Could you check a few things on this model? Use its own coordinates, in mm. Coordinates: 2 decimals unless noted, no trailing zeros. Write each loop counter-clockwise with the first axis right and the second up, starting at its lowest first coordinate (ties: lowest second). Pieces come first, ordered by that corner, then holes.
Item 1: I want a section at C-C on y = -323.5. Please give me the cut outline in (x, z), then the cut area to 3 significant figures.
Item 2: If I drill on probe 1 along Y at (x, z) = (-621, 1.3); probe 2 along X at (y, z) = (-349, 1.55); probe 3 along X at (y, z) = (-261, 1.55), over which ranges is the centre line in solid material (lowest first)?
Item 3: I want a section at A-A on z = 0.9. Please give me the cut outline in (x, y), then the cut area to 3 significant figures.
Item 4: I want a section at B-B on y = -208.5. Please give me the cut outline in (x, z), then the cut area to 3 significant figures.
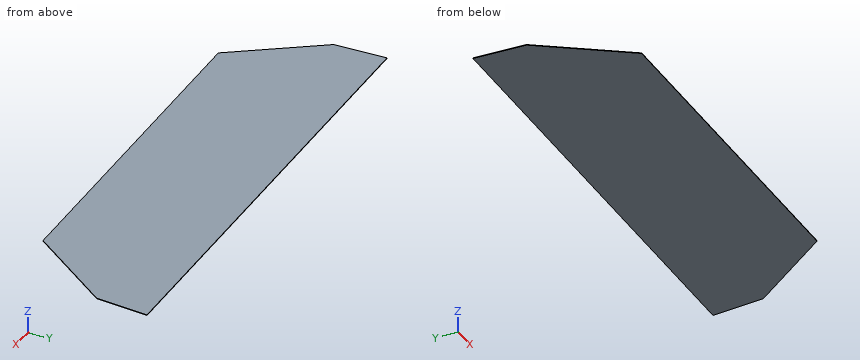
Autodesk Inventor part; units mm, degrees
ref_plane "YZ Plane" through (0, 0, 0) normal (1, 0, 0) x (0, 1, 0)
ref_plane "XZ Plane" through (0, 0, 0) normal (0, 1, 0) x (-1, 0, 0)
ref_plane "XY Plane" through (0, 0, 0) normal (0, 0, 1) x (1, 0, 0)
sketch "Sketch1" plane through (0, 0, 0) normal (0, 0, 1) x (1, 0, 0)
  line L0 (-760, -450) -> (760, -450)
  line L1 (760, -450) -> (760, 0)
  line L2 (760, 0) -> (-760, 0)
  line L3 (-760, 0) -> (-760, -450)
  point P0 (0, 0)
  point P1 (0, 0)
  dimension "d0" = 450
  dimension "d1" = 1520
extrude "Plate1" add sketch "Sketch1" along normal blind 2
sketch "Sketch2" plane through (0, 0, 2) normal (0, 0, 1) x (1, 0, 0)
  line L0 (760, -450) -> (-760, -450)
  line L1 (760, 0) -> (760, -450)
  line L2 (-760, 0) -> (760, 0)
  line L3 (-760, -450) -> (-760, 0)
  line L4 (759.9, 0) -> (750, -171)
  line L5 (750, -171) -> (555, -450)
  line L6 (760, -450) -> (-760, -450)
  point P0 (0, 0)
  dimension "d3" = 0.1
  dimension "d8" = 10
  dimension "d9" = 171
  dimension "d10" = 205
extrude "Extrusion1" cut sketch "Sketch2" against normal through all contours L0 L5 L4 L2 L1
mirror "Mirror1" about plane through (0, 0, 0) normal (1, 0, 0) of "Extrusion1"
equation "\"d2\" = Thickness"
equation "\"BendReliefWidth\" = Thickness"
equation "\"BendReliefDepth\" = 0.5 * Thickness"
equation "\"CornerReliefSize\" = 4 * Thickness"
equation "\"MinimumRemnant\" = 2 * Thickness"
equation "\"TransitionRadius\" = BendRadius"
equation "\"JacobiRadiusSize\" = BendRadius"
equation "\"GapSize\" = Thickness"
properties part number "MSC 704 face 4" material "Stainless Steel"
Response values:
1. outline: (-643.41, 0) - (643.41, 0) - (643.41, 2) - (-643.41, 2) - close
1. area: 2,570 mm2
2. probe 1: y = -355.57 to 0
2. probe 2: x = -625.59 to 625.59
2. probe 3: x = -687.1 to 687.1
3. outline: (-759.9, 0) - (-750, -171) - (-555, -450) - (555, -450) - (750, -171) - (759.9, 0) - close
3. area: 622,000 mm2
4. outline: (-723.79, 0) - (723.79, 0) - (723.79, 2) - (-723.79, 2) - close
4. area: 2,900 mm2
